Part model, mm, in its own coordinate system. Face numbers are marked on the shaded views. Coordinates: 2 decimals unless noted, no trailing zeros. Order: outer loops, then holes, each group sorted by start corner. A loop starts at its lowest first (then second) coordinate and runs counter-clockwise, first axis right, second up.
1) Cut at D-D (z = 17). List the corners of the cut face in (x, y), and give its area (3 significant figures).
2) Wall check: L1, parallel to Z at x = 0, y = 10.8; L2, parallel to Y at x = 0.5, z = 17; L3, parallel to Y at x = -3.5, z = 8. Give the ranges that are in metal, low to high.
3) Cut at C-C (z = 10.5). List the corners of the cut face in (x, y).
4) Mould opens along X. For the marked faces 1, 2 and 3 say: +X half, -X half, draft (parallel to the pull), parting line (faces both ways), or undercut.
5) Cut at A-A (x = 0). List the corners of the cut face in (y, z).
6) Pin check, flat tips, straight feed: pin 1 Ø10 at (x, z) = (-2.5, 4) entering from +Y; pin 2 Ø10 at (x, y) = (-1, -1.5) entering from +Z; pin 3 Ø5 at (x, y) = (2, -6.5) entering from -Z; pin 4 Ø10 at (x, z) = (9.5, -28) entering from +Y. Stop position of each tip, or through.
7) Cut at B-B (y = 0). List the corners of the cut face in (x, z), and give its area (3 significant figures).
```python
from build123d import *

# Parameters (mm, degrees)
SKETCH1_R           = 13
BOSS_EXTRUDE1_DEPTH = 20
SKETCH2_R           = 10.05
CUT_EXTRUDE1_DEPTH  = 15
SKETCH3_R           = 4
BOSS_EXTRUDE2_DEPTH = 35
FILLET1_R           = 2
CHAMFER1_SIZE       = 1
FILLET2_R           = 1
SKETCH4_R           = 2.5
CUT_EXTRUDE2_DEPTH  = 20


with BuildPart() as part:
    # Sketch1 → Boss-Extrude1 (new body)
    with BuildSketch(Plane.XY):
        Circle(SKETCH1_R)
    extrude(amount=BOSS_EXTRUDE1_DEPTH)

    # Sketch2 → Cut-Extrude1 (cut)
    with BuildSketch(Plane.XY.offset(20)):
        Circle(SKETCH2_R)
    extrude(amount=-CUT_EXTRUDE1_DEPTH, mode=Mode.SUBTRACT)

    # Sketch3 → Boss-Extrude2 (add)
    with BuildSketch(Plane(origin=(0, 0, 0), x_dir=(-1, 0, 0), z_dir=(0, 0, -1))):
        Circle(SKETCH3_R)
    extrude(amount=BOSS_EXTRUDE2_DEPTH)

    # Fillet1
    fillet1_edges = [part.edges().sort_by_distance(p)[0] for p in [
        (-13, 0, 0),
        (4, 0, 0),
    ]]
    fillet(fillet1_edges, radius=FILLET1_R)

    # Chamfer1
    chamfer1_edges = [part.edges().sort_by_distance(p)[0] for p in [
        (4, 0, -35),
    ]]
    chamfer(chamfer1_edges, length=CHAMFER1_SIZE)

    # Fillet2
    fillet2_edges = [part.edges().sort_by_distance(p)[0] for p in [
        (-13, 0, 20),
    ]]
    fillet(fillet2_edges, radius=FILLET2_R)

    # Sketch4 → Cut-Extrude2 (cut, symmetric)
    with BuildSketch(Plane(origin=(0, 0, 0), x_dir=(1, 0, 0), z_dir=(0, 1, 0))):
        with Locations(Location((0, -10.5, 0), (0, 0, 270))):
            Circle(SKETCH4_R)
    extrude(amount=CUT_EXTRUDE2_DEPTH, both=True, mode=Mode.SUBTRACT)


solid = part.part
```
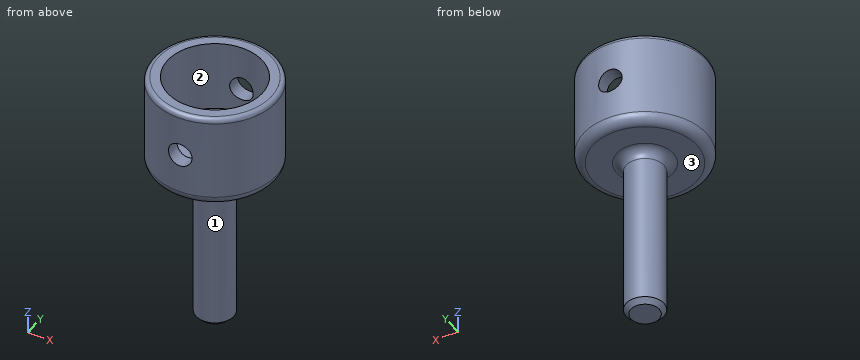
Geometry check:
1. outline: circle Ø26 at (0, 0); hole circle Ø20.1 at (0, 0)
1. area: 214 mm2
2. L1: z = 0 to 8, 13 to 20
2. L2: y = -12.99 to -10.04, 10.04 to 12.99
2. L3: y = -12.52 to -9.42, 9.42 to 12.52
3. outline: (-2.5, -12.76) - (-2.5, -9.73) arc R10.05 cw to (-2.5, 9.73) - (-2.5, 12.76) arc R13 ccw to start; (2.5, -12.76) arc R13 ccw to (2.5, 12.76) - (2.5, 9.73) arc R10.05 cw to (2.5, -9.73) - close
4. face 1: parting line
4. face 2: undercut
4. face 3: draft
5. outline: (-13, 2) arc R2 ccw to (-11, 0) - (-6, 0) arc R2 cw to (-4, -2) - (-4, -34) - (-3, -35) - (3, -35) - (4, -34) - (4, -2) arc R2 cw to (6, 0) - (11, 0) arc R2 ccw to (13, 2) - (13, 8) - (10.05, 8) - (10.05, 5) - (-10.05, 5) - (-10.05, 8) - (-13, 8) - close; (-13, 13) - (-10.05, 13) - (-10.05, 20) - (-12, 20) arc R1 ccw to (-13, 19) - close; (10.05, 13) - (13, 13) - (13, 19) arc R1 ccw to (12, 20) - (10.05, 20) - close
6. pin 1: stops at y = 13
6. pin 2: stops at z = 5
6. pin 3: stops at z = -0.95
6. pin 4: passes through
7. outline: (-13, 2) arc R2 ccw to (-11, 0) - (-6, 0) arc R2 cw to (-4, -2) - (-4, -34) - (-3, -35) - (3, -35) - (4, -34) - (4, -2) arc R2 cw to (6, 0) - (11, 0) arc R2 ccw to (13, 2) - (13, 19) arc R1 ccw to (12, 20) - (10.05, 20) - (10.05, 5) - (-10.05, 5) - (-10.05, 20) - (-12, 20) arc R1 ccw to (-13, 19) - close
7. area: 497 mm2
